Part model, mm, in its own coordinate system. Face numbers are marked on the shaded views. A direction names the side the tool comes from. Give positions to 0.01 mm unless a question says otherwise; leave off trailing zeros. Loops run counter-clockwise (first coordinate to the right, second up) from the corner with the lowest first, then second, coordinate; pieces in that order, holes last. Notation, with made-up numbers: M -23.5,30.5 L -12.5,30.5 A24 ccw -12.5,45.5 Z; hole C 37,-22.75 d6. An arc over 180 degrees is marked long. Answer in a Markdown table with one row per item.
from build123d import *

# Parameters (mm, degrees)
F0_W     = 600
F0_H     = 600
F1_DEPTH = 18
F2_W     = 18
F2_H     = 600
F3_DEPTH = 250
F4_W     = 18
F4_H     = 600
F5_DEPTH = 250


with BuildPart() as f1:
    # F0 (on Front) → F1 (new body)
    with BuildSketch(Plane.XZ):
        Rectangle(F0_W, F0_H)
    extrude(amount=F1_DEPTH)

    # F2 (on Front) → F3 (join)
    with BuildSketch(Plane.XZ):
        with Locations((-309, 0)):
            Rectangle(F2_W, F2_H)
    extrude(amount=F3_DEPTH)

    # F4 (on Front) → F5 (join)
    with BuildSketch(Plane.XZ):
        with Locations((309, 0)):
            Rectangle(F4_W, F4_H)
    extrude(amount=F5_DEPTH)


solid = f1.part
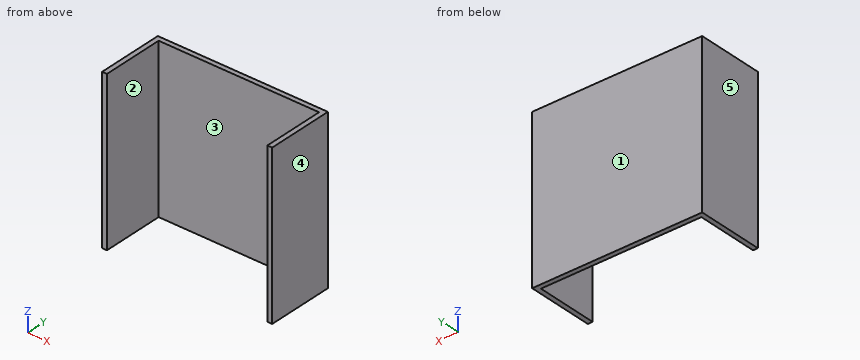
(1) Saw through at B-B (z = 231). Write the cut outline in (x, y).
Recorded:
| item | result |
|---|---|
| outline | M -318,-250 L -300,-250 L -300,-18 L 300,-18 L 300,-250 L 318,-250 L 318,0 L -318,0 Z |
(2) Pull direction X, two halves, no side cores. Call the marked faces 3, 4 and 5: +X half, -X half, draft (parallel to the pull), parting line (faces both ways), or undercut.
Recorded:
| item | result |
|---|---|
| face 3 | undercut |
| face 4 | +X half |
| face 5 | -X half |
(3) Saw through at C-C (x = -219.5). Write the cut outline in (y, z), plus the area to 3 significant figures.
Recorded:
| item | result |
|---|---|
| outline | M -18,-300 L 0,-300 L 0,300 L -18,300 Z |
| area | 10,800 mm^2 |
(4) Which spindle directions (+Z, -Z, +X, -X, +Y, -Y) get a long thin tool onto all of the face, cutting with end or side? Do the marked faces 1 and 2. Say none if no direction does.
Recorded:
| item | result |
|---|---|
| face 1 | +Z, -Z, +X, -X, +Y |
| face 2 | +Z, -Z, -Y |
(5) Saw through at A-A (y = -201). Write the cut outline in (x, z), plus the area to 3 significant figures.
Recorded:
| item | result |
|---|---|
| outline | M -318,-300 L -300,-300 L -300,300 L -318,300 Z; M 300,-300 L 318,-300 L 318,300 L 300,300 Z |
| area | 21,600 mm^2 |
(6) Drill centre lines: line 1 along X through (y, z) = (-50, 219.5); line 2 along Y through (x, z) = (214, -59.5). Where is each one in solid material? Low to high.
Recorded:
| item | result |
|---|---|
| line 1 | x = -318 to -300, 300 to 318 |
| line 2 | y = -18 to 0 |
